Here's how the part is built. I have some questions about the finished solid (model axes, mm). A direction names the side the tool comes from. Round coordinates to 2 decimals unless told otherwise and drop trailing zeros. Write each loop counter-clockwise with the first axis right and the second up, starting at its lowest first coordinate (ties: lowest second). Pieces come first, ordered by that corner, then holes. Notation, with made-up numbers: (84, -21) -> (110, -21) arc R7 cw to (110, -17) -> close; hole circle Ø3 at (89.25, -16.75). An arc over 180 degrees is marked (long way). Answer as CSV lines item,"result".
```python
from build123d import *

# Parameters (mm, degrees)
BOSS_EXTRUDE1_DEPTH = 176
SKETCH2_R           = 4
CUT_EXTRUDE1_DEPTH  = 90
SKETCH3_R           = 4
CUT_EXTRUDE2_DEPTH  = 12


with BuildPart() as part:
    # Sketch1 → Boss-Extrude1 (new body)
    with BuildSketch(Plane(origin=(0, 0, 0), x_dir=(0, 0, -1), z_dir=(1, 0, 0))):
        with BuildLine():
            Line((11, 53), (-11, 53))
            Line((-11, 53), (-11, -53))
            Line((-11, -53), (11, -53))
            Line((11, -53), (11, 15))
            ThreePointArc((11, 15), (12.757359313, 19.242640687), (17, 21))
            Line((17, 21), (24, 21))
            Line((24, 21), (24, 53))
            Line((24, 53), (11, 53))
        make_face()
    extrude(amount=BOSS_EXTRUDE1_DEPTH)

    # Sketch2 → Cut-Extrude1 (cut, symmetric)
    with BuildSketch(Plane(origin=(0, 0, -11), x_dir=(-1, 0, 0), z_dir=(0, 0, -1))):
        with Locations(Location((-69, 41, 0), (0, 0, 90))):
            Circle(SKETCH2_R)
        with Locations(Location((-107, 41, 0), (0, 0, 90))):
            Circle(SKETCH2_R)
        with Locations(Location((-68.580611035, -5, 0), (0, 0, 90))):
            Circle(SKETCH2_R)
        with Locations(Location((-107.419388965, -5, 0), (0, 0, 90))):
            Circle(SKETCH2_R)
    extrude(amount=CUT_EXTRUDE1_DEPTH, both=True, mode=Mode.SUBTRACT)

    # Sketch3 → Cut-Extrude2 (cut)
    with BuildSketch(Plane(origin=(0, 53, 0), x_dir=(1, 0, 0), z_dir=(0, 1, 0))):
        with Locations(Location((32, 6.5, 0), (0, 0, 270))):
            Circle(SKETCH3_R)
        with Locations(Location((144, 6.5, 0), (0, 0, 90))):
            Circle(SKETCH3_R)
    extrude(amount=-CUT_EXTRUDE2_DEPTH, mode=Mode.SUBTRACT)


solid = part.part
```
1. For pin 1 Ø20.5 at (x, y) = (54.5, -3) entering from -Z; pin 2 Ø5.5 at (x, z) = (62, -19) entering from -Y; pin 3 Ø4 at (x, z) = (32.5, -7) entering from +Y, each with a flat end and sliding along its axis, tell me the tip position at first contact or that it passes through.
Numbers:
pin 1,"stops at z = -11"
pin 2,"stops at y = 20.95"
pin 3,"stops at y = 41"
2. If I drill on line 1 (X direction, y = -5, z = -6); line 2 (X direction, y = 41, z = 9); line 3 (Y direction, x = 69, z = -6.5), over which ranges is the centre line in solid material (lowest first)?
Numbers:
line 1,"x = 0 to 64.58, 72.58 to 103.42, 111.42 to 176"
line 2,"x = 0 to 65, 73 to 103, 111 to 176"
line 3,"y = -53 to -8.98, -1.02 to 37, 45 to 53"
3. On a 3-axis mill with a long thin cutter (end or side, diameter ignored), from which of +Z, -Z, +X, -X, +Y, -Y can I reach the whole of each face in a straight line? I mean faces 1 (the face through (144, 41, -6)), 2 (the face through (72.547, -5.521, -0.154)), 3 (the face through (87, 21, -20)). Say none if no direction works.
Numbers:
face 1,"+Y"
face 2,"+Z, -Z"
face 3,"-Z, +X, -X, -Y"
4. Suppose I cut it at B-B on x = 18. Please give me the cut outline in (y, z), and give its area (3 significant figures).
Numbers:
outline,"(-53, -11) -> (15, -11) arc R6 cw to (21, -17) -> (21, -24) -> (53, -24) -> (53, 11) -> (-53, 11) -> close"
area,"2,760 mm^2"
5. Suppose I cut it at C-C on z = -6.5. Please give me the cut outline in (x, y), and give its area (3 significant figures).
Numbers:
outline,"(0, -53) -> (176, -53) -> (176, 53) -> (148, 53) -> (148, 41) -> (140, 41) -> (140, 53) -> (36, 53) -> (36, 41) -> (28, 41) -> (28, 53) -> (0, 53) -> close; hole circle Ø8 at (68.58, -5); hole circle Ø8 at (69, 41); hole circle Ø8 at (107, 41); hole circle Ø8 at (107.42, -5)"
area,"18,300 mm^2"
6. Suppose I cut it at D-D on y = -20. Please give me the cut outline in (x, z), and give its area (3 significant figures).
Numbers:
outline,"(0, -11) -> (176, -11) -> (176, 11) -> (0, 11) -> close"
area,"3,870 mm^2"
7. If we mould it in two halves opening along Z, with no side actions, what happens to faces 4 (the face through (32, 41, -7)), 5 (the face through (87, -53, 0)), 6 (the face through (87, 37, -24))? For each: released by +Z, released by -Z, zero draft, split by the parting line, or undercut.
Numbers:
face 4,"undercut"
face 5,"zero draft"
face 6,"released by -Z"
8. Suppose I cut it at A-A on y = -5. Please give me the cut outline in (x, z).
Numbers:
outline,"(0, -11) -> (64.58, -11) -> (64.58, 11) -> (0, 11) -> close; (72.58, -11) -> (103.42, -11) -> (103.42, 11) -> (72.58, 11) -> close; (111.42, -11) -> (176, -11) -> (176, 11) -> (111.42, 11) -> close"
